Source: CAD feature listing. Evaluate the final solid. Frame: model axes, mm. Face numbers are marked on the shaded views. Give positions to 0.01 mm unless a question says otherwise; leave off trailing zeros. Order: outer loops, then holes, each group sorted by start corner. A loop starts at its lowest first (then second) coordinate and runs counter-clockwise, first axis right, second up.
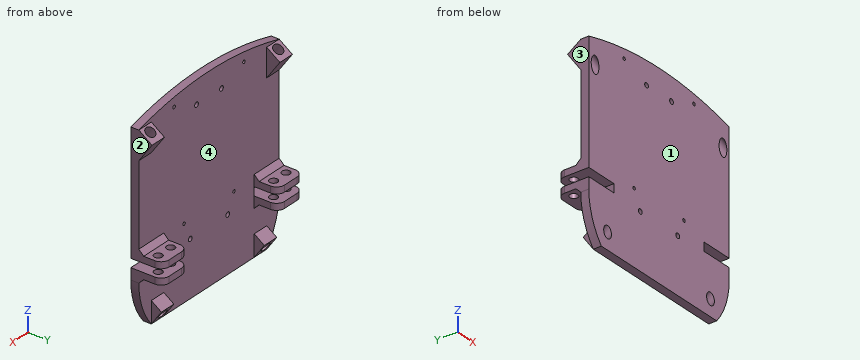
```python
from build123d import *

# Parameters (mm, degrees)
BOSS_EXTRUDE1_DEPTH      = 2.5
BOSS_EXTRUDE2_DEPTH      = 10
SKETCH3_R                = 3.1
CUT_EXTRUDE1_DEPTH       = 97.926231277
BOSS_EXTRUDE3_DEPTH      = 10
SKETCH5_R                = 3.1
CUT_EXTRUDE2_DEPTH       = 73.924932584
SKETCH6_W                = 5.175957564
SKETCH6_H                = 5
CUT_EXTRUDE3_DEPTH       = 113.454585159
SKETCH7_W                = 20.15
SKETCH7_H                = 0.476848187
BOSS_EXTRUDE4_DEPTH      = 5
SKETCH7_3_W              = 20.15
SKETCH7_3_H              = 0.476848187
CUT_EXTRUDE4_DEPTH       = 5
SKETCH8_W                = 4
SKETCH8_H                = 15
BOSS_EXTRUDE5_DEPTH      = 20
SKETCH9_R                = 2.5
CUT_EXTRUDE5_DEPTH       = 13.3
FILLET1_R                = 5
CHAMFER1_SIZE            = 3
FILLET1_OF_MIRROR2_R     = 5
CHAMFER1_OF_MIRROR2_SIZE = 3
BOSS_EXTRUDE6_DEPTH      = 5
SKETCH11_R               = 1
CUT_EXTRUDE6_DEPTH       = 6
SKETCH12_R               = 1.5
CUT_EXTRUDE7_DEPTH       = 21
CUT_EXTRUDE8_DEPTH       = 6


with BuildPart() as part:
    # Sketch1 → Boss-Extrude1 (new body, symmetric)
    with BuildSketch(Plane(origin=(-32.81203924, 33.9517387, -54.90733973), x_dir=(-1, 0, 0), z_dir=(0, -1, 0))):
        Polygon((57.454585159, 35), (-55, 35), (-55, 0.15), (-34.85, 0.15), (-34.85, -5.15), (-55, -5.15), (-55, -85), (57.454585159, -85), (57.454585159, -4.673151813), (37.304585159, -4.673151813), (37.304585159, 0.626848187), (57.454585159, 0.626848187), align=None)
    extrude(amount=BOSS_EXTRUDE1_DEPTH, both=True)

    # Sketch2 → Boss-Extrude2 (add)
    with BuildSketch(Plane.ZY.offset(90.266624399)):
        Polygon((7.48223475, 36.4517387), (19.180938343, 44.643259143), (24.916702706, 36.4517387), align=None)
    boss_extrude2 = extrude(amount=-BOSS_EXTRUDE2_DEPTH)

    # Sketch3 → Cut-Extrude1 (cut, through all)
    with BuildSketch(Plane(origin=(0, 23.699275736, 33.846073404), x_dir=(1, 0, 0), z_dir=(0, 0.573576436, 0.819152044))):
        with Locations((-85.266624399, 19.56788273)):
            Circle(SKETCH3_R)
    cut_extrude1 = extrude(amount=-CUT_EXTRUDE1_DEPTH, mode=Mode.SUBTRACT)

    # Sketch4 → Boss-Extrude3 (add)
    with BuildSketch(Plane(origin=(-70.266624399, 0, 0), x_dir=(0, 0, -1), z_dir=(1, 0, 0))):
        Polygon((76.559676692, 36.4517387), (80.950923398, 42.723088931), (89.90733973, 36.4517387), align=None)
    boss_extrude3 = extrude(amount=-BOSS_EXTRUDE3_DEPTH)

    # Sketch5 → Cut-Extrude2 (cut, through all)
    with BuildSketch(Plane(origin=(0, 66.702115647, -46.70532419), x_dir=(1, 0, 0), z_dir=(0, 0.819152044, -0.573576436))):
        with Locations((-75.266624399, 47.224033141)):
            Circle(SKETCH5_R)
    cut_extrude2 = extrude(amount=-CUT_EXTRUDE2_DEPTH, mode=Mode.SUBTRACT)

    # Mirror1: Boss-Extrude2, Cut-Extrude1, Boss-Extrude3, Cut-Extrude2 across plane
    add(boss_extrude2.mirror(Plane.ZY.offset(34.03933182)))
    add(cut_extrude1.mirror(Plane.ZY.offset(34.03933182)), mode=Mode.SUBTRACT)
    add(boss_extrude3.mirror(Plane.ZY.offset(34.03933182)))
    add(cut_extrude2.mirror(Plane.ZY.offset(34.03933182)), mode=Mode.SUBTRACT)

    # Sketch6 → Cut-Extrude3 (cut, through all)
    with BuildSketch(Plane.ZY.offset(90.266624399)):
        with Locations((27.504681488, 33.9517387)):
            Rectangle(SKETCH6_W, SKETCH6_H)
    extrude(amount=-CUT_EXTRUDE3_DEPTH, mode=Mode.SUBTRACT)

    # Sketch7 → Boss-Extrude4 (add)
    with BuildSketch(Plane(origin=(0, 36.4517387, 0), x_dir=(1, 0, 0), z_dir=(0, 1, 0))):
        with Locations((-80.191624399, 55.295763824)):
            Rectangle(SKETCH7_W, SKETCH7_H)
    boss_extrude4 = extrude(amount=-BOSS_EXTRUDE4_DEPTH)

    # Sketch7<3> → Cut-Extrude4 (cut)
    with BuildSketch(Plane(origin=(0, 36.4517387, 0), x_dir=(1, 0, 0), z_dir=(0, 1, 0))):
        with Locations((-80.191624399, 49.995763823)):
            Rectangle(SKETCH7_3_W, SKETCH7_3_H)
    cut_extrude4 = extrude(amount=-CUT_EXTRUDE4_DEPTH, mode=Mode.SUBTRACT)

    # Sketch8 → Boss-Extrude5 (add)
    with BuildSketch(Plane.ZY.offset(90.266624399)):
        with Locations((-57.05733973, 43.9517387)):
            Rectangle(SKETCH8_W, SKETCH8_H)
        with Locations((-47.75733973, 43.9517387)):
            Rectangle(SKETCH8_W, SKETCH8_H)
    boss_extrude5 = extrude(amount=-BOSS_EXTRUDE5_DEPTH)

    # Sketch9 → Cut-Extrude5 (cut)
    with BuildSketch(Plane(origin=(0, 0, -59.05733973), x_dir=(-1, 0, 0), z_dir=(0, 0, -1))):
        with Locations((75.266624399, 44.643259143)):
            Circle(SKETCH9_R)
        with Locations((85.266624399, 44.643259143)):
            Circle(SKETCH9_R)
    cut_extrude5 = extrude(amount=-CUT_EXTRUDE5_DEPTH, mode=Mode.SUBTRACT)

    # Fillet1
    fillet1_edges = [part.edges().sort_by_distance(p)[0] for p in [
        (-70.266624399, 51.4517387, -57.05733973),
        (-90.266624399, 51.4517387, -57.05733973),
        (-70.266624399, 51.4517387, -47.75733973),
        (-90.266624399, 51.4517387, -47.75733973),
    ]]
    fillet(fillet1_edges, radius=FILLET1_R)

    # Chamfer1
    chamfer1_edges = [part.edges().sort_by_distance(p)[0] for p in [
        (-80.266624399, 36.4517387, -59.05733973),
        (-80.266624399, 36.4517387, -45.75733973),
    ]]
    chamfer(chamfer1_edges, length=CHAMFER1_SIZE)

    # Mirror2: Boss-Extrude4, Cut-Extrude4, Boss-Extrude5, Cut-Extrude5 across plane
    add(boss_extrude4.mirror(Plane.ZY.offset(34.03933182)))
    add(cut_extrude4.mirror(Plane.ZY.offset(34.03933182)), mode=Mode.SUBTRACT)
    add(boss_extrude5.mirror(Plane.ZY.offset(34.03933182)))
    add(cut_extrude5.mirror(Plane.ZY.offset(34.03933182)), mode=Mode.SUBTRACT)

    # Fillet1 of Mirror2
    fillet1_of_mirror2_edges = [part.edges().sort_by_distance(p)[0] for p in [
        (2.18796076, 51.4517387, -57.05733973),
        (22.18796076, 51.4517387, -57.05733973),
        (2.18796076, 51.4517387, -47.75733973),
        (22.18796076, 51.4517387, -47.75733973),
    ]]
    fillet(fillet1_of_mirror2_edges, radius=FILLET1_OF_MIRROR2_R)

    # Chamfer1 of Mirror2
    chamfer1_of_mirror2_edges = [part.edges().sort_by_distance(p)[0] for p in [
        (12.18796076, 36.4517387, -59.05733973),
        (12.18796076, 36.4517387, -45.75733973),
    ]]
    chamfer(chamfer1_of_mirror2_edges, length=CHAMFER1_OF_MIRROR2_SIZE)

    # Sketch10 → Boss-Extrude6 (add)
    with BuildSketch(Plane(origin=(0, 36.4517387, 0), x_dir=(1, 0, 0), z_dir=(0, 1, 0))):
        with BuildLine():
            Line((-90.266624399, -24.916702706), (22.18796076, -24.916702706))
            ThreePointArc((22.18796076, -24.916702706), (-34.03933182, -32.584076644), (-90.266624399, -24.916702706))
        make_face()
    extrude(amount=-BOSS_EXTRUDE6_DEPTH)

    # Sketch11 → Cut-Extrude6 (cut, through all)
    with BuildSketch(Plane(origin=(0, 36.4517387, 0), x_dir=(1, 0, 0), z_dir=(0, 1, 0))):
        with Locations((-54.03933182, 44.951248934)):
            Circle(SKETCH11_R)
        with Locations((-14.03933182, 44.951248934)):
            Circle(SKETCH11_R)
        with Locations((-6.03933182, -25.048751066)):
            Circle(SKETCH11_R)
        with Locations((-62.03933182, -25.048751066)):
            Circle(SKETCH11_R)
    extrude(amount=-CUT_EXTRUDE6_DEPTH, mode=Mode.SUBTRACT)

    # Sketch12 → Cut-Extrude7 (cut, through all)
    with BuildSketch(Plane.XZ.offset(-31.4517387)):
        with Locations((-19.03933182, -55.87359945)):
            Circle(SKETCH12_R)
        with Locations((-24.03933182, 18.12640055)):
            Circle(SKETCH12_R)
        with Locations((-49.03933182, -55.87359945)):
            Circle(SKETCH12_R)
        with Locations((-44.03933182, 18.12640055)):
            Circle(SKETCH12_R)
    extrude(amount=-CUT_EXTRUDE7_DEPTH, mode=Mode.SUBTRACT)

    # Sketch13 → Cut-Extrude8 (cut, through all)
    with BuildSketch(Plane(origin=(0, 36.4517387, 0), x_dir=(1, 0, 0), z_dir=(0, 1, 0))):
        with BuildLine():
            ThreePointArc((-90.266624399, 62.05733973), (-87.690854406, 76.852799337), (-80.266624399, 89.90733973))
            Line((-80.266624399, 89.90733973), (-90.266624399, 89.90733973))
            Line((-90.266624399, 89.90733973), (-90.266624399, 62.05733973))
        make_face()
        with BuildLine():
            ThreePointArc((22.18796076, 62.05733973), (19.612190767, 76.852799337), (12.18796076, 89.90733973))
            Line((12.18796076, 89.90733973), (22.18796076, 89.90733973))
            Line((22.18796076, 89.90733973), (22.18796076, 62.05733973))
        make_face()
    extrude(amount=-CUT_EXTRUDE8_DEPTH, mode=Mode.SUBTRACT)


solid = part.part
```
1) Section query A-A, the plane y = 48.5. Return the cut outline in (x, z), and give its area (3 significant figures).
Report:
outline: (-89.83, -59.06) - (-70.71, -59.06) - (-70.71, -55.06) - (-89.83, -55.06) - close; (-89.83, -49.76) - (-70.71, -49.76) - (-70.71, -45.76) - (-89.83, -45.76) - close; (2.63, -59.06) - (21.75, -59.06) - (21.75, -55.06) - (2.63, -55.06) - close; (2.63, -49.76) - (21.75, -49.76) - (21.75, -45.76) - (2.63, -45.76) - close
area: 306 mm2
2) Section query B-B, the plane z = -4.5. Return the cut outline in (x, y), and give its area (3 significant figures).
Report:
outline: (-90.27, 31.45) - (22.19, 31.45) - (22.19, 36.45) - (-90.27, 36.45) - close
area: 562 mm2
3) Draft query along X for the marked faces 1, 2, 3 and 4. Return one class per face: +X half, -X half, draft (parallel to the pull), parting line (faces both ways), or undercut.
Report:
face 1: draft
face 2: +X half
face 3: -X half
face 4: undercut
4) Section query C-C, the plane y = 34.75. Count the separate pieces of the cut face and the enclosed holes in it, and give its area (3 significant figures).
Report:
separate pieces: 1
enclosed holes: 12
area: 12,900 mm2
5) Material intervals for L1, parallel to Z at x = 9, y = 37.75; L2, parallel to Y at x = -31, z = -73; L3, parallel to Z at x = 7.5, y = 39.75, sorted ascending.
Report:
L1: z = -88.05 to -87.15, -81.01 to -77.47, -60.76 to -55.06, -49.76 to -44.06
L2: y = 31.45 to 36.45
L3: z = -81.72 to -78.87, -59.06 to -55.06, -49.76 to -45.76
6) Section query D-D, the plane x = -68.5. Return the cut outline in (y, z).
Report:
outline: (31.45, -89.91) - (36.45, -89.91) - (36.45, 29.74) - (31.45, 29.74) - close
7) Pin query (flat end, axial travel): pin 1 (1.8 mm diameter, centred on x = -44.04, z = 18.13, fed in from +Y); pin 2 (4.5 mm diameter, centred on x = -85.27, y = 44.64, fed in from +Z); pin 3 (2 mm diameter, centred on x = -70, y = 48, fed in from +Z); pin 4 (6 mm diameter, centred on x = -77.5, y = 40.5, fed in from +Z). Return the tip coordinate at first contact, or that it passes through.
Report:
pin 1: passes through
pin 2: stops at z = 20.76
pin 3: stops at z = -45.76
pin 4: stops at z = 22.89
